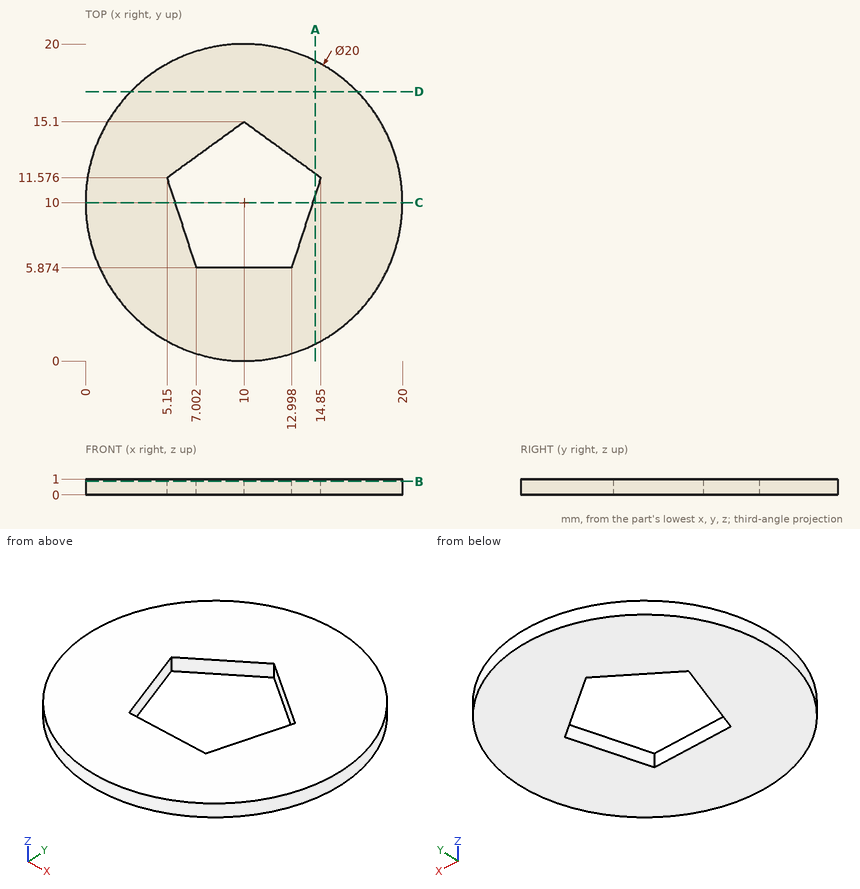
Could you check a few things on this drawing? It's one solid part, dimensions in mm from its lowest x, y, z. Round coordinates to 2 decimals unless told otherwise and drop trailing zeros. Write each loop counter-clockwise with the first axis right and the second up, starting at its lowest first coordinate (ties: lowest second). Pieces come first, ordered by that corner, then holes. Notation, with made-up numbers: M 14,-37 L 57,-37 A11 cw 57,-33 Z; hole C -40,23 d1. An arc over 180 degrees is marked long. Answer as CSV lines item,"result". Start each with the question number.
1. I need wall thicknesses on probe 1 along Y at (x, z) = (9.5, 0.5) (1 decimal); probe 2 along X at (y, z) = (14, 0.6) (1 decimal); probe 3 along Y at (x, z) = (7.75, 0.6) (1 decimal). Which ranges of each line are inside material? Lowest first, please.
2. Suppose I cut it at A-A on x = 14.5. Write out the boundary of the cut face in (y, z).
3. Suppose I cut it at D-D on y = 17. Write out the boundary of the cut face in (x, z), then the cut area to 3 significant figures.
4. Suppose I cut it at B-B on z = 0.85. Write out the boundary of the cut face in (x, y).
5. Suppose I cut it at C-C on y = 10. Write out the boundary of the cut face in (x, z).
Check result:
1,probe 1,"y = 0 to 5.9, 14.7 to 20"
1,probe 2,"x = 0.8 to 8.5, 11.5 to 19.2"
1,probe 3,"y = 0.3 to 5.9, 13.5 to 19.7"
2,outline,"M 1.07,0 L 10.5,0 L 10.5,1 L 1.07,1 Z; M 11.83,0 L 18.93,0 L 18.93,1 L 11.83,1 Z"
3,outline,"M 2.86,0 L 17.14,0 L 17.14,1 L 2.86,1 Z"
3,area,"14.3 mm2"
4,outline,"C 10,10 d20; hole M 5.15,11.58 L 7,5.87 L 13,5.87 L 14.85,11.58 L 10,15.1 Z"
5,outline,"M 0,0 L 5.66,0 L 5.66,1 L 0,1 Z; M 14.34,0 L 20,0 L 20,1 L 14.34,1 Z"
